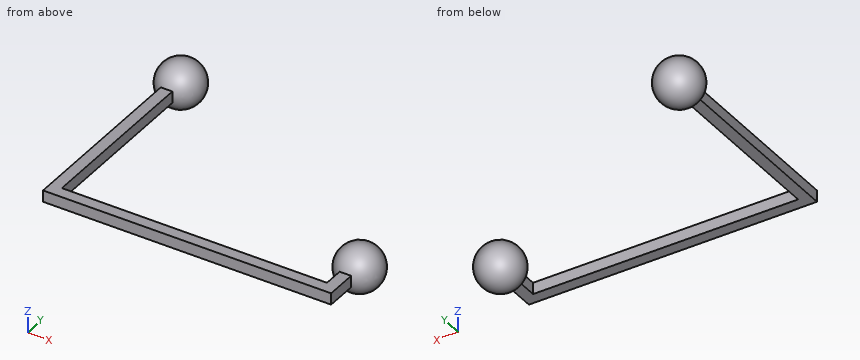
```python
from build123d import *

# Parameters (mm, degrees)
BOSS_EXTRUDE1_DEPTH = 3.175


with BuildPart() as part:
    # Sketch1 → Boss-Extrude1 (new body)
    with BuildSketch(Plane.XY):
        Polygon((0, 0), (79.375, 0), (79.375, 8.638996592), (76.2, 8.638996592), (76.2, 3.175), (3.175, 3.175), (3.175, 50.8), (0, 50.8), align=None)
    extrude(amount=BOSS_EXTRUDE1_DEPTH)

    # Sketch2 → Revolve1 (revolve)
    with BuildSketch(Plane.XY.offset(1.5875)):
        with BuildLine():
            Line((1.5875, 50.598361062), (1.5875, 63.298361062))
            ThreePointArc((1.5875, 63.298361062), (7.9375, 56.948361062), (1.5875, 50.598361062))
        make_face()
    revolve(axis=Axis((1.5875, 50.598361062, 1.5875), (0, 1, 0)))

    # Sketch3 → Revolve2 (revolve)
    with BuildSketch(Plane.XY.offset(1.5875)):
        with BuildLine():
            Line((77.7875, 21.137357655), (77.7875, 8.437357655))
            ThreePointArc((77.7875, 8.437357655), (84.1375, 14.787357655), (77.7875, 21.137357655))
        make_face()
    revolve(axis=Axis((77.7875, 21.137357655, 1.5875), (0, -1, 0)))


solid = part.part
```
Work out the finished part from the listing and answer in its coordinate system (mm). Round coordinates to 2 decimals unless told otherwise and drop trailing zeros. Loops run counter-clockwise (first coordinate to the right, second up) from the corner with the lowest first, then second, coordinate; pieces in that order, holes last.
(1) The part is cut by section B-B, the plane z = -1.75. Give the vertices of the cut face in (x, y), and give its area (3 significant figures).
Computed values:
outline: circle Ø10.8 at (1.59, 56.95); circle Ø10.8 at (77.79, 14.79)
area: 183 mm2
(2) Each of these flat-tipped pins is pushed along its axis until it touches: P1, Ø0.8, axis at x = 77.5, z = 2.5, coming from the +Y side; P2, Ø3.5, axis at y = 3.5, z = 1.5, coming from the +X side (3 decimals); P3, Ø4, axis at y = 26, z = 6, coming from the -X side; P4, Ø2.5, axis at x = 42.5, z = 2, coming from the +Y side (3 decimals). Where does it stop, or does it pass through?
Computed values:
P1: stops at y = 21.11
P2: stops at x = 79.375
P3: passes through
P4: stops at y = 3.175
(3) Find the intervals of material crossed by L1, parallel to X at y = 4.5, z = 0.5 (3 decimals); L2, parallel to Y at x = 40, z = 0.75 (3 decimals), in increasing order.
Computed values:
L1: x = 0 to 3.175, 76.2 to 79.375
L2: y = 0 to 3.175
(4) The part is cut by section C-C, the plane x = 5. Give the vertices of the cut face in (y, z) (1 decimal), and give its area (3 significant figures).
Computed values:
outline: (0, 0) - (3.2, 0) - (3.2, 3.2) - (0, 3.2) - close; circle Ø10.7 at (56.9, 1.6)
area: 100 mm2
(5) The part is cut by section A-A, the plane y = 15. Give the vertices of the cut face in (x, z) (1 decimal).
Computed values:
outline: (0, 0) - (3.2, 0) - (3.2, 3.2) - (0, 3.2) - close; circle Ø12.7 at (77.8, 1.6)
(6) The part is cut by section D-D, the plane y = 48.5. Give the vertices of the cut face in (x, z) (3 decimals), and give its area (3 significant figures).
Computed values:
outline: (0, 0) - (3.175, 0) - (3.175, 3.175) - (0, 3.175) - close
area: 10.1 mm2
